Input: part model. Units: mm. Frame: model coordinates. A direction names the side the tool comes from. Round coordinates to 2 decimals unless told otherwise and drop trailing zeros. Order: outer loops, then holes, each group sorted by start corner. A loop starts at its lowest first (then second) coordinate and runs counter-clockwise, first axis right, second up. Notation, with made-up numbers: (-8, 10.25) -> (15, 10.25) arc R36 ccw to (15, 49.25) -> close; hole circle Ø5 at (70.5, 35.5). An arc over 180 degrees is marked (long way). Use a Markdown table: item, result.
from build123d import *

# Parameters (mm, degrees)
CUT_EXTRUDE1_REACH = 21.05
SKETCH2_R          = 2.15265
SKETCH2_R_2        = 3.175
SKETCH3_R          = 0.396875
CUT_EXTRUDE2_DEPTH = 6.35


with BuildPart() as part:
    # Sketch1 → Revolve1 (revolve)
    with BuildSketch(Plane.XY):
        Polygon((-36.83, 19.05), (-6.35, 19.05), (-6.35, 0), (-20.447, 0), (-20.447, 6.35), (-14.097, 6.35), (-14.097, 12.7), (-36.83, 12.7), align=None)
    revolve(axis=Axis((0, 0, 0), (0, 1, 0)))

    # Sketch2 → Cut-Extrude1 (cut, up to next)
    with BuildSketch(Plane(origin=(0, 19.05, 0), x_dir=(1, 0, 0), z_dir=(0, 1, 0)), mode=Mode.PRIVATE) as cut_extrude1_sk1:
        with Locations((0, 30.48)):
            Circle(SKETCH2_R)
    cut_extrude1_tool1 = extrude(cut_extrude1_sk1.sketch, amount=-CUT_EXTRUDE1_REACH, mode=Mode.PRIVATE) & part.part
    add(cut_extrude1_tool1.solids().sort_by_distance((0, 19.05, -30.48))[0], mode=Mode.SUBTRACT)
    # Sketch2 → Cut-Extrude1 (cut, up to next)
    with BuildSketch(Plane(origin=(0, 19.05, 0), x_dir=(1, 0, 0), z_dir=(0, 1, 0)), mode=Mode.PRIVATE) as cut_extrude1_sk2:
        with Locations((11.664191018, 28.159848151)):
            Circle(SKETCH2_R)
    cut_extrude1_tool2 = extrude(cut_extrude1_sk2.sketch, amount=-CUT_EXTRUDE1_REACH, mode=Mode.PRIVATE) & part.part
    add(cut_extrude1_tool2.solids().sort_by_distance((11.664191, 19.05, -28.159848))[0], mode=Mode.SUBTRACT)
    # Sketch2 → Cut-Extrude1 (cut, up to next)
    with BuildSketch(Plane(origin=(0, 19.05, 0), x_dir=(1, 0, 0), z_dir=(0, 1, 0)), mode=Mode.PRIVATE) as cut_extrude1_sk3:
        with Locations((21.552614691, 21.552614691)):
            Circle(SKETCH2_R)
    cut_extrude1_tool3 = extrude(cut_extrude1_sk3.sketch, amount=-CUT_EXTRUDE1_REACH, mode=Mode.PRIVATE) & part.part
    add(cut_extrude1_tool3.solids().sort_by_distance((21.552615, 19.05, -21.552615))[0], mode=Mode.SUBTRACT)
    # Sketch2 → Cut-Extrude1 (cut, up to next)
    with BuildSketch(Plane(origin=(0, 19.05, 0), x_dir=(1, 0, 0), z_dir=(0, 1, 0)), mode=Mode.PRIVATE) as cut_extrude1_sk4:
        with Locations((28.159848151, 11.664191018)):
            Circle(SKETCH2_R)
    cut_extrude1_tool4 = extrude(cut_extrude1_sk4.sketch, amount=-CUT_EXTRUDE1_REACH, mode=Mode.PRIVATE) & part.part
    add(cut_extrude1_tool4.solids().sort_by_distance((28.159848, 19.05, -11.664191))[0], mode=Mode.SUBTRACT)
    # Sketch2 → Cut-Extrude1 (cut, up to next)
    with BuildSketch(Plane(origin=(0, 19.05, 0), x_dir=(1, 0, 0), z_dir=(0, 1, 0)), mode=Mode.PRIVATE) as cut_extrude1_sk5:
        with Locations((30.48, 0)):
            Circle(SKETCH2_R)
    cut_extrude1_tool5 = extrude(cut_extrude1_sk5.sketch, amount=-CUT_EXTRUDE1_REACH, mode=Mode.PRIVATE) & part.part
    add(cut_extrude1_tool5.solids().sort_by_distance((30.48, 19.05, 0))[0], mode=Mode.SUBTRACT)
    # Sketch2 → Cut-Extrude1 (cut, up to next)
    with BuildSketch(Plane(origin=(0, 19.05, 0), x_dir=(1, 0, 0), z_dir=(0, 1, 0)), mode=Mode.PRIVATE) as cut_extrude1_sk6:
        with Locations((28.159848151, -11.664191018)):
            Circle(SKETCH2_R)
    cut_extrude1_tool6 = extrude(cut_extrude1_sk6.sketch, amount=-CUT_EXTRUDE1_REACH, mode=Mode.PRIVATE) & part.part
    add(cut_extrude1_tool6.solids().sort_by_distance((28.159848, 19.05, 11.664191))[0], mode=Mode.SUBTRACT)
    # Sketch2 → Cut-Extrude1 (cut, up to next)
    with BuildSketch(Plane(origin=(0, 19.05, 0), x_dir=(1, 0, 0), z_dir=(0, 1, 0)), mode=Mode.PRIVATE) as cut_extrude1_sk7:
        with Locations((21.552614691, -21.552614691)):
            Circle(SKETCH2_R)
    cut_extrude1_tool7 = extrude(cut_extrude1_sk7.sketch, amount=-CUT_EXTRUDE1_REACH, mode=Mode.PRIVATE) & part.part
    add(cut_extrude1_tool7.solids().sort_by_distance((21.552615, 19.05, 21.552615))[0], mode=Mode.SUBTRACT)
    # Sketch2 → Cut-Extrude1 (cut, up to next)
    with BuildSketch(Plane(origin=(0, 19.05, 0), x_dir=(1, 0, 0), z_dir=(0, 1, 0)), mode=Mode.PRIVATE) as cut_extrude1_sk8:
        with Locations((11.664191019, -28.159848151)):
            Circle(SKETCH2_R)
    cut_extrude1_tool8 = extrude(cut_extrude1_sk8.sketch, amount=-CUT_EXTRUDE1_REACH, mode=Mode.PRIVATE) & part.part
    add(cut_extrude1_tool8.solids().sort_by_distance((11.664191, 19.05, 28.159848))[0], mode=Mode.SUBTRACT)
    # Sketch2 → Cut-Extrude1 (cut, up to next)
    with BuildSketch(Plane(origin=(0, 19.05, 0), x_dir=(1, 0, 0), z_dir=(0, 1, 0)), mode=Mode.PRIVATE) as cut_extrude1_sk9:
        with Locations((0, -30.48)):
            Circle(SKETCH2_R)
    cut_extrude1_tool9 = extrude(cut_extrude1_sk9.sketch, amount=-CUT_EXTRUDE1_REACH, mode=Mode.PRIVATE) & part.part
    add(cut_extrude1_tool9.solids().sort_by_distance((0, 19.05, 30.48))[0], mode=Mode.SUBTRACT)
    # Sketch2 → Cut-Extrude1 (cut, up to next)
    with BuildSketch(Plane(origin=(0, 19.05, 0), x_dir=(1, 0, 0), z_dir=(0, 1, 0)), mode=Mode.PRIVATE) as cut_extrude1_sk10:
        with Locations((-11.664191018, -28.159848151)):
            Circle(SKETCH2_R)
    cut_extrude1_tool10 = extrude(cut_extrude1_sk10.sketch, amount=-CUT_EXTRUDE1_REACH, mode=Mode.PRIVATE) & part.part
    add(cut_extrude1_tool10.solids().sort_by_distance((-11.664191, 19.05, 28.159848))[0], mode=Mode.SUBTRACT)
    # Sketch2 → Cut-Extrude1 (cut, up to next)
    with BuildSketch(Plane(origin=(0, 19.05, 0), x_dir=(1, 0, 0), z_dir=(0, 1, 0)), mode=Mode.PRIVATE) as cut_extrude1_sk11:
        with Locations((-21.552614691, -21.552614691)):
            Circle(SKETCH2_R)
    cut_extrude1_tool11 = extrude(cut_extrude1_sk11.sketch, amount=-CUT_EXTRUDE1_REACH, mode=Mode.PRIVATE) & part.part
    add(cut_extrude1_tool11.solids().sort_by_distance((-21.552615, 19.05, 21.552615))[0], mode=Mode.SUBTRACT)
    # Sketch2 → Cut-Extrude1 (cut, up to next)
    with BuildSketch(Plane(origin=(0, 19.05, 0), x_dir=(1, 0, 0), z_dir=(0, 1, 0)), mode=Mode.PRIVATE) as cut_extrude1_sk12:
        with Locations((-28.159848151, -11.664191018)):
            Circle(SKETCH2_R)
    cut_extrude1_tool12 = extrude(cut_extrude1_sk12.sketch, amount=-CUT_EXTRUDE1_REACH, mode=Mode.PRIVATE) & part.part
    add(cut_extrude1_tool12.solids().sort_by_distance((-28.159848, 19.05, 11.664191))[0], mode=Mode.SUBTRACT)
    # Sketch2 → Cut-Extrude1 (cut, up to next)
    with BuildSketch(Plane(origin=(0, 19.05, 0), x_dir=(1, 0, 0), z_dir=(0, 1, 0)), mode=Mode.PRIVATE) as cut_extrude1_sk13:
        with Locations((-30.48, 0)):
            Circle(SKETCH2_R)
    cut_extrude1_tool13 = extrude(cut_extrude1_sk13.sketch, amount=-CUT_EXTRUDE1_REACH, mode=Mode.PRIVATE) & part.part
    add(cut_extrude1_tool13.solids().sort_by_distance((-30.48, 19.05, 0))[0], mode=Mode.SUBTRACT)
    # Sketch2 → Cut-Extrude1 (cut, up to next)
    with BuildSketch(Plane(origin=(0, 19.05, 0), x_dir=(1, 0, 0), z_dir=(0, 1, 0)), mode=Mode.PRIVATE) as cut_extrude1_sk14:
        with Locations((-28.159848151, 11.664191018)):
            Circle(SKETCH2_R)
    cut_extrude1_tool14 = extrude(cut_extrude1_sk14.sketch, amount=-CUT_EXTRUDE1_REACH, mode=Mode.PRIVATE) & part.part
    add(cut_extrude1_tool14.solids().sort_by_distance((-28.159848, 19.05, -11.664191))[0], mode=Mode.SUBTRACT)
    # Sketch2 → Cut-Extrude1 (cut, up to next)
    with BuildSketch(Plane(origin=(0, 19.05, 0), x_dir=(1, 0, 0), z_dir=(0, 1, 0)), mode=Mode.PRIVATE) as cut_extrude1_sk15:
        with Locations((-21.552614691, 21.552614691)):
            Circle(SKETCH2_R)
    cut_extrude1_tool15 = extrude(cut_extrude1_sk15.sketch, amount=-CUT_EXTRUDE1_REACH, mode=Mode.PRIVATE) & part.part
    add(cut_extrude1_tool15.solids().sort_by_distance((-21.552615, 19.05, -21.552615))[0], mode=Mode.SUBTRACT)
    # Sketch2 → Cut-Extrude1 (cut, up to next)
    with BuildSketch(Plane(origin=(0, 19.05, 0), x_dir=(1, 0, 0), z_dir=(0, 1, 0)), mode=Mode.PRIVATE) as cut_extrude1_sk16:
        with Locations((-11.664191018, 28.159848151)):
            Circle(SKETCH2_R)
    cut_extrude1_tool16 = extrude(cut_extrude1_sk16.sketch, amount=-CUT_EXTRUDE1_REACH, mode=Mode.PRIVATE) & part.part
    add(cut_extrude1_tool16.solids().sort_by_distance((-11.664191, 19.05, -28.159848))[0], mode=Mode.SUBTRACT)
    # Sketch2 → Cut-Extrude1 (cut, up to next)
    with BuildSketch(Plane(origin=(0, 19.05, 0), x_dir=(1, 0, 0), z_dir=(0, 1, 0)), mode=Mode.PRIVATE) as cut_extrude1_sk17:
        with Locations((-17.272, 0)):
            Circle(SKETCH2_R_2)
    cut_extrude1_tool17 = extrude(cut_extrude1_sk17.sketch, amount=-CUT_EXTRUDE1_REACH, mode=Mode.PRIVATE) & part.part
    add(cut_extrude1_tool17.solids().sort_by_distance((-17.272, 19.05, 0))[0], mode=Mode.SUBTRACT)

    # Sketch3 → Cut-Extrude2 (cut)
    with BuildSketch(Plane.XZ):
        with Locations((0, 16.51)):
            Circle(SKETCH3_R)
        with Locations((3.220941216, 16.192764979)):
            Circle(SKETCH3_R)
        with Locations((6.318103468, 15.253251082)):
            Circle(SKETCH3_R)
        with Locations((9.172464547, 13.727563299)):
            Circle(SKETCH3_R)
        with Locations((11.674332957, 11.674332957)):
            Circle(SKETCH3_R)
        with Locations((13.727563299, 9.172464547)):
            Circle(SKETCH3_R)
        with Locations((15.253251082, 6.318103468)):
            Circle(SKETCH3_R)
        with Locations((16.192764979, 3.220941216)):
            Circle(SKETCH3_R)
        with Locations((16.51, 0)):
            Circle(SKETCH3_R)
        with Locations((16.192764979, -3.220941216)):
            Circle(SKETCH3_R)
        with Locations((15.253251082, -6.318103468)):
            Circle(SKETCH3_R)
        with Locations((13.727563299, -9.172464547)):
            Circle(SKETCH3_R)
        with Locations((11.674332957, -11.674332957)):
            Circle(SKETCH3_R)
        with Locations((9.172464547, -13.727563299)):
            Circle(SKETCH3_R)
        with Locations((6.318103468, -15.253251082)):
            Circle(SKETCH3_R)
        with Locations((3.220941217, -16.192764979)):
            Circle(SKETCH3_R)
        with Locations((0, -16.51)):
            Circle(SKETCH3_R)
        with Locations((-3.220941216, -16.192764979)):
            Circle(SKETCH3_R)
        with Locations((-6.318103468, -15.253251082)):
            Circle(SKETCH3_R)
        with Locations((-9.172464547, -13.727563299)):
            Circle(SKETCH3_R)
        with Locations((-11.674332957, -11.674332957)):
            Circle(SKETCH3_R)
        with Locations((-13.727563299, -9.172464547)):
            Circle(SKETCH3_R)
        with Locations((-15.253251082, -6.318103468)):
            Circle(SKETCH3_R)
        with Locations((-16.192764979, -3.220941216)):
            Circle(SKETCH3_R)
        with Locations((-16.51, 0)):
            Circle(SKETCH3_R)
        with Locations((-16.192764979, 3.220941216)):
            Circle(SKETCH3_R)
        with Locations((-15.253251082, 6.318103468)):
            Circle(SKETCH3_R)
        with Locations((-13.727563299, 9.172464547)):
            Circle(SKETCH3_R)
        with Locations((-11.674332957, 11.674332957)):
            Circle(SKETCH3_R)
        with Locations((-9.172464547, 13.727563299)):
            Circle(SKETCH3_R)
        with Locations((-6.318103468, 15.253251082)):
            Circle(SKETCH3_R)
        with Locations((-3.220941216, 16.192764979)):
            Circle(SKETCH3_R)
    extrude(amount=-CUT_EXTRUDE2_DEPTH, mode=Mode.SUBTRACT)


solid = part.part
1) Ray query, probe 1 along Z at (x, y) = (29, 17.25); probe 2 along Z at (x, y) = (0, 4); probe 3 along X at (y, z) = (14.5, -1). Return the intervals inside material, ascending.
Answer key:
| item | result |
|---|---|
| probe 1 | z = -22.7 to -13.65, -9.68 to -1.56, 1.56 to 9.68, 13.65 to 22.7 |
| probe 2 | z = -20.45 to -16.91, -16.11 to -6.35, 6.35 to 16.11, 16.91 to 20.45 |
| probe 3 | x = -36.82 to -32.39, -28.57 to -20.29, -14.26 to -6.27, 6.27 to 28.57, 32.39 to 36.82 |
2) Cut plane B-B on y = 4.5. State how many separate pieces and enclosed holes the cut face has, and give its area (3 significant figures).
Answer key:
| item | result |
|---|---|
| separate pieces | 1 |
| enclosed holes | 33 |
| area | 1,170 mm^2 |
3) Draft query along Z for faces 4 (the face through (10.08, 15.92, 26.7)), 5 (the face through (16.226, 3.219, -12.442)), 6 (the face through (-29.87, 15.92, 12.97)), 7 (the face through (-5, 0, 5)). Return one class per face: released by +Z, released by -Z, zero draft, split by the parting line, or undercut.
Answer key:
| item | result |
|---|---|
| face 4 | undercut |
| face 5 | split by the parting line |
| face 6 | undercut |
| face 7 | zero draft |
4) Cut plane A-A on z = -22.5. Return loops of the section in (x, y), and give its area (3 significant figures).
Answer key:
| item | result |
|---|---|
| outline | (-29.16, 12.7) -> (-23.49, 12.7) -> (-23.49, 19.05) -> (-29.16, 19.05) -> close; (-19.62, 12.7) -> (19.62, 12.7) -> (19.62, 19.05) -> (-19.62, 19.05) -> close; (23.49, 12.7) -> (29.16, 12.7) -> (29.16, 19.05) -> (23.49, 19.05) -> close |
| area | 321 mm^2 |
5) Set-up query: faces 1 (the face through (-14.244, 15.919, -0.954)), 2 (the face through (-1.59, 15.92, 29.03)), 3 (the face through (-9, 6.35, -13)). Return all of +Z, -Z, +X, -X, +Y, -Y with unobstructed straight access to the full face (end or side cutting, diameter ignored); none if empty.
Answer key:
| item | result |
|---|---|
| face 1 | +Y |
| face 2 | +Y, -Y |
| face 3 | none |
6) Contact query for flat-ended pins moving along their axis: P1, Ø5, axis at y = 15.5, z = 19, coming from the -X side; P2, Ø5, axis at y = 7.5, z = 23, coming from the +X side; P3, Ø5, axis at x = 28.16, z = -11.66, coming from the -Y side; P4, Ø1.5, axis at y = 13.5, z = 25, coming from the +X side. Output: stop coordinate, or through.
Answer key:
| item | result |
|---|---|
| P1 | stops at x = -32.93 |
| P2 | passes through |
| P3 | stops at y = 12.7 |
| P4 | stops at x = 27.72 |
7) Cut plane C-C on y = 9.75. Return loops of the section in (x, z), and give its area (3 significant figures).
Answer key:
| item | result |
|---|---|
| outline | circle Ø28.19 at (0, 0); hole circle Ø12.7 at (0, 0) |
| area | 498 mm^2 |
